```python
from build123d import *

# Parameters (mm, degrees)
F1_DEPTH = 2.54
F2_R     = 0.508


with BuildPart() as f1:
    # F0 (on Top) → F1 (new body)
    with BuildSketch(Plane.XY):
        Polygon((-22.761848, -17.692075), (0, 0), (0, 6.550886), (-92.096252, 49.455902), align=None)
        Polygon((-85.790934, 45.117378), (-0.635, 5.445659), (-0.635, 1.485886), (-1.476617, 0.826895), (-22.88023, -15.809466), align=None, mode=Mode.SUBTRACT)
    extrude(amount=F1_DEPTH)

    # F2
    f2_edges = [f1.edges().sort_by_distance(p)[0] for p in [
        (-57.42905, 15.881913, 2.54),
        (-11.380924, -8.846038, 2.54),
        (-46.048126, 28.003394, 2.54),
        (-46.048126, 28.003394, 0),
        (-57.42905, 15.881913, 0),
    ]]
    fillet(f2_edges, radius=F2_R)


solid = f1.part
```
Read the model definition and answer for the solid it produces. Units are mm, in the model's axes. A direction names the side the tool comes from. Give positions to 0.01 mm unless a question says otherwise; leave off trailing zeros. Loops run counter-clockwise (first coordinate to the right, second up) from the corner with the lowest first, then second, coordinate; pieces in that order, holes last.
Item 1: For faces 4 (the flat face through (-0.635, 3, 1)), 5 (the flat face through (-45.4, 27.7, 1.3)), determine the directions among +Z, -Z, +X, -X, +Y, -Y from which every point of the face is accessible in a straight line to the end or side of a thin tool.
Item 2: This flat-tipped pin is pushed along its axis until it touches: pin 1 Ø1.5 at (x, z) = (-34.5, 0.5) entering from +Y. Where does it stop, or does it pass through?
Item 3: The part is cut by section A-A (z = 1.35). Write down the section's boundary in (x, y) (3 decimals).
Item 4: Find the intervals of material crossed by line 1 along Y through (x, z) = (-27.5, 0.3); line 2 along X through (y, z) = (15.5, 0.6); line 3 along X through (y, z) = (35, 1.1), in increasing order.
Item 5: The mould has two halves that part along Y. Classify faces 1 (the cylindrical face through (-46.65, 28.12, 0.15)), 2 (the flat face through (-53.9, 14.23, 1.25)), 3 (the cylindrical face through (-56.84, 15.52, 2.39)): released by +Y, released by -Y, zero draft, split by the parting line, or undercut.
Taken from the geometry:
1. face 4: +Z, -Z
1. face 5: +Z, -Z, +X, +Y
2. pin 1: stops at y = 22.97
3. outline: (-92.096, 49.456) - (-22.762, -17.692) - (0, 0) - (0, 6.551) - close; hole (-85.791, 45.117) - (-22.88, -15.809) - (-1.477, 0.827) - (-0.635, 1.486) - (-0.635, 5.446) - close
4. line 1: y = -13.04 to -11.34, 17.96 to 19.31
4. line 2: x = -57.03 to -55.21, -22.22 to -19.21
4. line 3: x = -77.17 to -75.34, -64.07 to -61.07
5. face 1: released by +Y
5. face 2: undercut
5. face 3: released by -Y
